Can you work these out from the drawing? Everything is in mm from the part's minimum corner. Round coordinates to 2 decimals unless told otherwise and drop trailing zeros. Write each loop counter-clockwise with the first axis right and the second up, starting at its lowest first coordinate (ties: lowest second). Pieces come first, ordered by that corner, then holes. Notation, with made-up numbers: (-26, 20.25) -> (5, 20.25) arc R19 ccw to (5, 26.25) -> close; hole circle Ø10 at (-4.75, -7). An arc over 180 degrees is marked (long way). Put each result on its own line as item: value. Start each with the question number.
1. Suppose I cut it at B-B (y = 52.5). Please give me the cut outline in (x, z).
2. Suppose I cut it at A-A (z = 16.25). Please give me the cut outline in (x, y).
3. We'd pull the mould along Y, two halves only. Please class the marked faces 1, 2 and 3: +Y half, -Y half, draft (parallel to the pull), parting line (faces both ways), or undercut.
4. Suppose I cut it at C-C (x = 207). Please give me the cut outline in (y, z).
5. I need wall thicknesses on probe 1 along X at (y, z) = (37, 8.75); probe 2 along Y at (x, z) = (195, 5.5); probe 3 along Z at (x, y) = (151.5, 21). Which ranges of each line are inside material? Lowest first, please. Write a range as from..to.
6. For pin 1 (10 mm diameter, centred on x = 64, y = 20, fed in from +Z), with a flat end and sliding along its axis, tell me the tip position at first contact or that it passes through.
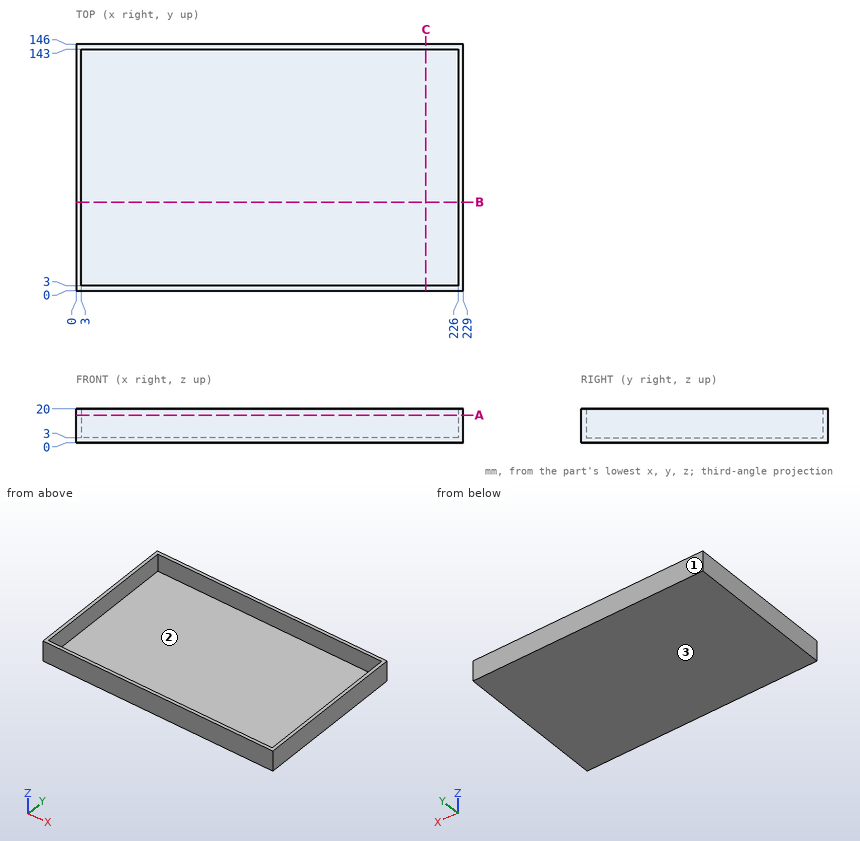
Verdict:
1. outline: (0, 0) -> (229, 0) -> (229, 20) -> (226, 20) -> (226, 3) -> (3, 3) -> (3, 20) -> (0, 20) -> close
2. outline: (0, 0) -> (229, 0) -> (229, 146) -> (0, 146) -> close; hole (3, 3) -> (226, 3) -> (226, 143) -> (3, 143) -> close
3. face 1: +Y half
3. face 2: undercut
3. face 3: draft
4. outline: (0, 0) -> (146, 0) -> (146, 20) -> (143, 20) -> (143, 3) -> (3, 3) -> (3, 20) -> (0, 20) -> close
5. probe 1: x = 0..3, 226..229
5. probe 2: y = 0..3, 143..146
5. probe 3: z = 0..3
6. pin 1: stops at z = 3
